The listing builds one solid part. Answer for the finished solid, in the listing's coordinates (mm). Face numbers are marked on the shaded views. Round coordinates to 2 decimals unless told otherwise and drop trailing zeros. Write each loop counter-clockwise with the first axis right and the second up, starting at its lowest first coordinate (ties: lowest second). Pieces come first, ordered by that corner, then holes.
(1) A cutting plane is placed at B-B, the plane x = -80. Give the vertices of the cut face in (y, z).
(2) Find the intervals of material crossed by probe 1 along Z at (x, y) = (-60, -51.1); probe 2 along Y at (x, z) = (-20, -0.35); probe 3 along Y at (x, z) = (-60, 0), in increasing order.
(3) A cutting plane is placed at A-A, the plane x = -60. Give the vertices of the cut face in (y, z), and give its area (3 significant figures).
(4) A cutting plane is placed at C-C, the plane y = -36. Give the vertices of the cut face in (x, z), and give its area (3 significant figures).
(5) The mould has two halves that part along Y. Classify the marked faces 1 and 2: +Y half, -Y half, draft (parallel to the pull), parting line (faces both ways), or undercut.
(6) Each of these flat-tipped pins is pushed along its axis until it touches: pin 1 Ø2 at (x, z) = (-113, 0) entering from -Y; pin 2 Ø1 at (x, z) = (-63, 11.5) entering from +Y; pin 3 Ø3.5 at (y, z) = (-51, 17.5) entering from +X. Where does it stop, or does it pass through?
(7) A cutting plane is placed at D-D, the plane x = -120. Give the vertices of the cut face in (y, z), and give its area (3 significant figures).
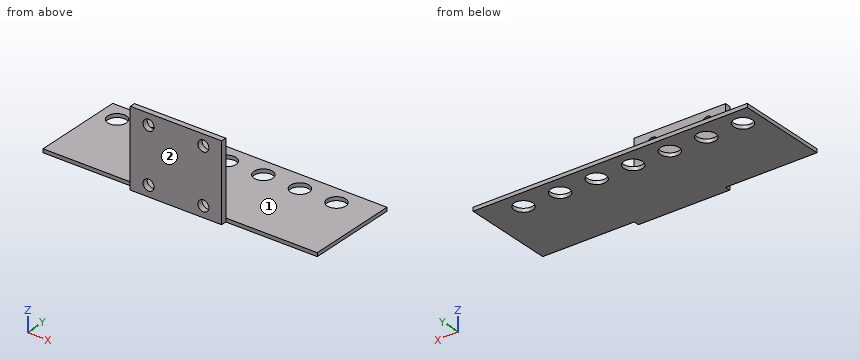
Autodesk Fusion 360 part; units mm, degrees
sketch "Sketch1" plane through (0, 0, 0) normal (0, 0, 1) x (1, 0, 0)
  line L0 (0, 0) -> (-150, 0)
  line L1 (-150, 0) -> (-150, -50)
  line L2 (-150, -50) -> (0, -50)
  line L3 (0, -50) -> (0, 0)
  dimension "d1" = 150
extrude "Extrude1" add sketch "Sketch1" along normal blind 1
sketch "Sketch2" plane through (0, -50, 0) normal (0, -1, 0) x (1, 0, 0)
  line L0 (-150, 0) -> (0, 0)
  line L1 (0, 0) -> (0, 1)
  line L2 (0, 1) -> (-150, 1)
  line L3 (-150, 1) -> (-150, 0)
  line L4 (-100, 0) -> (-50, 0)
  line L5 (-50, 0) -> (-50, 1)
  line L6 (-50, 1) -> (-100, 1)
  line L7 (-100, 1) -> (-100, 0)
  dimension "d4" = 50
extrude "Extrude2" add sketch "Sketch2" along normal blind 1 contours L0 L2 L4 L5 L6 L7
extrude "Extrude3" add 1 faces at (-83.3333, -51, 0.6667) along direction (0, -1, 0) blind 2
sketch "Sketch3" plane through (0, 0, 1) normal (0, 0, 1) x (-1, 0, 0)
  line L0 (0, 50) -> (0, 0)
  line L1 (0, 0) -> (150, 0)
  line L2 (150, 0) -> (150, 50)
  line L3 (150, 50) -> (100, 50)
  line L4 (100, 50) -> (100, 53)
  line L5 (100, 53) -> (50, 53)
  line L6 (50, 53) -> (50, 50)
  line L7 (50, 50) -> (0, 50)
  line L8 (100, 50) -> (50, 50)
  line L9 (50, 50) -> (50, 53)
  line L10 (50, 53) -> (100, 53)
  line L11 (100, 53) -> (100, 50)
extrude "Extrude4" add sketch "Sketch3" along normal blind 40 contours L4 L5 L6 L8 L9 L10 L11
extrude "Extrude5" add 1 faces at (-83.3333, -16.6667, 0) along direction (0, 0, -1) blind 1
sketch "Sketch4" plane through (0, -53, 0) normal (0, -1, 0) x (1, 0, 0)
  line L0 (-100, 41) -> (-100, -1)
  line L1 (-100, -1) -> (-50, -1)
  line L2 (-50, -1) -> (-50, 41)
  line L3 (-50, 41) -> (-100, 41)
  circle A0 centre (-60, 35) radius 3
  circle A1 centre (-60, 5) radius 3
  dimension "d13" = 6
  dimension "d14" = 6
sketch "Sketch5" plane through (0, -53, 0) normal (0, -1, 0) x (1, 0, 0)
  circle A0 centre (-90, 35) radius 3
  circle A1 centre (-90, 5) radius 3
  dimension "d15" = 6
  dimension "d16" = 6
extrude "Extrude6" cut sketch "Sketch4" sketch "Sketch5" against normal blind 15 contours A0 | A1 of sketch 2
sketch "Sketch6" plane through (0, 0, -1) normal (0, 0, -1) x (1, 0, 0)
  line L0 (0, 0) -> (0, 50)
  line L1 (0, 50) -> (-50, 50)
  line L2 (-50, 50) -> (-50, 53)
  line L3 (-50, 53) -> (-100, 53)
  line L4 (-100, 53) -> (-100, 50)
  line L5 (-100, 50) -> (-150, 50)
  line L6 (-150, 50) -> (-150, 0)
  line L7 (-150, 0) -> (0, 0)
  circle A0 centre (-140, 10) radius 5.1
  circle A1 centre (-120, 10) radius 5.1
  circle A2 centre (-100, 10) radius 5.1
  circle A3 centre (-80, 10) radius 5.1
  circle A4 centre (-60, 10) radius 5.1
  circle A5 centre (-40, 10) radius 5.1
  circle A6 centre (-20, 10) radius 5.1
  dimension "d19" = 10.2
  dimension "d20" = 10.2
  dimension "d21" = 10.2
  dimension "d22" = 10.2
  dimension "d23" = 10.2
  dimension "d24" = 10.2
  dimension "d25" = 10.2
extrude "Extrude7" cut sketch "Sketch6" against normal blind 10 contours A0 | A1 | A2 | A3 | A4 | A5 | A6
Solutions:
1. outline: (-53, -1) - (-15.1, -1) - (-15.1, 1) - (-50, 1) - (-50, 41) - (-53, 41) - close; (-4.9, -1) - (0, -1) - (0, 1) - (-4.9, 1) - close
2. probe 1: z = -1 to 2, 8 to 32, 38 to 41
2. probe 2: y = -50 to -15.1, -4.9 to 0
2. probe 3: y = -53 to -15.1, -4.9 to 0
3. outline: (-53, -1) - (-15.1, -1) - (-15.1, 1) - (-50, 1) - (-50, 2) - (-53, 2) - close; (-53, 8) - (-50, 8) - (-50, 32) - (-53, 32) - close; (-53, 38) - (-50, 38) - (-50, 41) - (-53, 41) - close; (-4.9, -1) - (0, -1) - (0, 1) - (-4.9, 1) - close
3. area: 170 mm2
4. outline: (-150, -1) - (0, -1) - (0, 1) - (-150, 1) - close
4. area: 300 mm2
5. face 1: draft
5. face 2: -Y half
6. pin 1: stops at y = -50
6. pin 2: stops at y = -50
6. pin 3: stops at x = -50
7. outline: (-50, -1) - (-15.1, -1) - (-15.1, 1) - (-50, 1) - close; (-4.9, -1) - (0, -1) - (0, 1) - (-4.9, 1) - close
7. area: 79.6 mm2
